Autodesk Inventor part; units mm, degrees
ref_plane "YZ Plane" through (0, 0, 0) normal (1, 0, 0) x (0, 1, 0)
ref_plane "XZ Plane" through (0, 0, 0) normal (0, 1, 0) x (-1, 0, 0)
ref_plane "XY Plane" through (0, 0, 0) normal (0, 0, 1) x (1, 0, 0)
sketch "スケッチ1" plane through (0, 0, 0) normal (1, 0, 0) x (0, 1, 0)
  circle A0 centre (19.5992, 5.9415) radius 1.7
  circle A1 centre (-9.4008, 5.9415) radius 1.7
  line L0 (-2.2068, 22.1678) -> (-6.2315, 30.9988)
  arc A2 (-6.2315, 30.9988) -> (5.9783, 33.4275) centre (5.0992, 5.9415) ccw
  line L1 (5.6395, 23.7285) -> (-2.2068, 22.1678)
  circle A3 centre (5.0992, 5.9415) radius 7.75
  line L2 (5.9783, 33.4275) -> (5.6395, 23.7285)
  point P0 (0, 0)
extrude "押し出し1" add sketch "スケッチ1" along normal blind 2.5
properties part number "belt_liner_v2_3DP_P-2-F" material "ABS プラスチック"
Geometry check sheet. Reference: the model listing, model coordinates, mm. A direction names the side the tool comes from. Give positions to 0.01 mm unless a question says otherwise; leave off trailing zeros. Write each loop counter-clockwise with the first axis right and the second up, starting at its lowest first coordinate (ties: lowest second). Pieces come first, ordered by that corner, then holes. Notation, with made-up numbers: (-2, 53) - (24, 53) arc R20 cw to (24, 73) - close; hole circle Ø11 at (39, 4.25). An arc over 180 degrees is marked (long way). Put each result on its own line as item: value.
1. Sectioned sample at D-D, the plane x = 0.7. Enter the section's corners in (y, z).
Ans:
outline: (-6.23, 31) arc R27.5 ccw (long way) to (5.98, 33.43) - (5.64, 23.73) - (-2.21, 22.17) - close; hole circle Ø3.4 at (-9.4, 5.94); hole circle Ø15.5 at (5.1, 5.94); hole circle Ø3.4 at (19.6, 5.94)
2. Go/stop test with flat-tipped pins: pin 1 (1 mm diameter, centred on x = 1.5, z = -6.5, fed in from -Y); pin 2 (1 mm diameter, centred on x = 1.5, y = -14.5, fed in from -Z); pin 3 (1.5 mm diameter, centred on x = 2, z = -1, fed in from -Y). Record where each tip stops, or that it passes through.
Ans:
pin 1: stops at y = -19.67
pin 2: stops at z = -13.84
pin 3: stops at y = -21.69
3. Set-up check for faces 4 (the flat face through (1.23, 1.77, 22.96)), 5 (the cylindrical face through (1.23, -10.65, 4.79)): record each of +Z, -Z, +X, -X, +Y, -Y from which the full face is reachable in a straight line by a thin tool's end or side.
Ans:
face 4: +Z, +X, -X
face 5: +X, -X
4. Sectioned sample at A-A, the plane z = 23. Enter the section's corners in (x, y), plus the area to 3 significant figures.
Ans:
outline: (0, -16.47) - (2.5, -16.47) - (2.5, -2.59) - (0, -2.59) - close; (0, 1.98) - (2.5, 1.98) - (2.5, 26.67) - (0, 26.67) - close
area: 96.4 mm²
5. Draft check along Z on faces 1 (the flat face through (2.5, 11, 0)), 2 (the flat face through (1.23, -4.19, 26.52)), 3 (the cylindrical face through (1.2, 17.9, 5.9)). Enter one of: +Z half, -Z half, draft (parallel to the pull), parting line (faces both ways), or undercut.
Ans:
face 1: draft
face 2: +Z half
face 3: undercut
6. Sectioned sample at B-B, the plane y = 7.5. Enter the section's corners in (x, z).
Ans:
outline: (0, -21.45) - (2.5, -21.45) - (2.5, -1.43) - (0, -1.43) - close; (0, 13.31) - (2.5, 13.31) - (2.5, 33.34) - (0, 33.34) - close
7. Thickness scan on line 1 (Z direction, x = 1.75, y = 5); line 2 (Y direction, x = 0.45, z = 25); line 3 (Y direction, x = 2.1, z = 27.5). Record the ranges inside material, lowest first.
Ans:
line 1: z = -21.56 to -1.81, 13.69 to 23.6
line 2: y = -14.73 to -3.5, 5.68 to 24.92
line 3: y = -11.97 to -4.64, 5.77 to 22.17
8. Sectioned sample at C-C, the plane z = 7. Enter the section's corners in (x, y).
Ans:
outline: (0, -22.38) - (2.5, -22.38) - (2.5, -10.73) - (0, -10.73) - close; (0, -8.07) - (2.5, -8.07) - (2.5, -2.58) - (0, -2.58) - close; (0, 12.78) - (2.5, 12.78) - (2.5, 18.27) - (0, 18.27) - close; (0, 20.93) - (2.5, 20.93) - (2.5, 32.58) - (0, 32.58) - close
